Input: part model. Units: mm. Frame: model coordinates. A direction names the side the tool comes from. Give positions to 0.01 mm unless a question says otherwise; leave off trailing zeros. Loops run counter-clockwise (first coordinate to the right, second up) from the corner with the lowest first, then second, coordinate; pieces in that order, holes last. Notation, with made-up numbers: (-28.75, 65.25) - (-13.75, 65.25) arc R15 cw to (-13.75, 86.25) - close; hole circle Ø9 at (26, 39.25). An arc over 180 degrees is marked (long way). Answer as a JSON object with one key per item and string values. Group by question number.
(1) Access query for faces 1 (the flat face through (62.5, 22, 0)), 2 (the flat face through (-30, 4, 0)). Directions: +Z, -Z, +X, -X, +Y, -Y. A direction counts if a zero-diameter tool reaches every point of the face in a straight line with its end or side. Return the directions, or none.
(2) Pin query (flat end, axial travel): P1, Ø8.5, axis at x = 10, z = -4.5, coming from the +Y side; P2, Ø15, axis at x = 41.5, z = -8, coming from the +Y side. Return the tip coordinate at first contact, or that it passes through.
(3) Material intervals for L1, parallel to X at y = 7.5, z = 19.5; L2, parallel to Z at x = 12.5, y = 9.5; L3, parallel to X at y = 16, z = -3.5, sorted ascending.
(4) Section query A-A (y = 27.5). Return loops of the section in (x, z).
(5) Section query D-D (x = -30). Return loops of the section in (y, z).
(6) Section query B-B (z = 18). Return loops of the section in (x, y), plus the area to 3 significant figures.
(7) Section query C-C (x = 48). Return loops of the section in (y, z).
(8) Mould query, pull axis X, two halves, no side actions, for faces 3 (the flat face through (-62.5, 22, 0)), 4 (the flat face through (-1, 22, 23)), 5 (the flat face through (15, 8.5, 0)), 6 (the flat face through (59.5, 25, 0)). Classes: +X half, -X half, draft (parallel to the pull), parting line (faces both ways), or undercut.
```python
from build123d import *

# Parameters (mm, degrees)
SKETCH1_W           = 119
SKETCH1_H           = 40
BOSS_EXTRUDE1_DEPTH = 4
SKETCH2_W           = 125
SKETCH2_H           = 46
SKETCH2_W_2         = 119
SKETCH2_H_2         = 40
BOSS_EXTRUDE2_DEPTH = 44
SKETCH3_W           = 58.2
SKETCH3_H           = 40
BOSS_EXTRUDE3_DEPTH = 3
SKETCH4_W           = 28
SKETCH4_H           = 40
BOSS_EXTRUDE4_DEPTH = 1.5


with BuildPart() as part:
    # Sketch1 → Boss-Extrude1 (new body)
    with BuildSketch(Plane(origin=(0, 0, 0), x_dir=(1, 0, 0), z_dir=(0, 1, 0))):
        Rectangle(SKETCH1_W, SKETCH1_H)
    extrude(amount=BOSS_EXTRUDE1_DEPTH)

    # Sketch2 → Boss-Extrude2 (add)
    with BuildSketch(Plane(origin=(0, 0, 0), x_dir=(1, 0, 0), z_dir=(0, 1, 0))):
        Rectangle(SKETCH2_W, SKETCH2_H)
        Rectangle(SKETCH2_W_2, SKETCH2_H_2, mode=Mode.SUBTRACT)
    extrude(amount=BOSS_EXTRUDE2_DEPTH)

    # Sketch3 → Boss-Extrude3 (add)
    with BuildSketch(Plane(origin=(0, 4, 0), x_dir=(1, 0, 0), z_dir=(0, 1, 0))):
        with Locations((30.4, 0)):
            Rectangle(SKETCH3_W, SKETCH3_H)
    extrude(amount=BOSS_EXTRUDE3_DEPTH)

    # Sketch4 → Boss-Extrude4 (add)
    with BuildSketch(Plane(origin=(0, 7, 0), x_dir=(1, 0, 0), z_dir=(0, 1, 0))):
        with Locations((15.3, 0)):
            Rectangle(SKETCH4_W, SKETCH4_H)
    extrude(amount=BOSS_EXTRUDE4_DEPTH)


solid = part.part
```
Recorded:
{
 "1": {"face 1": "+Z, -Z, +X, +Y, -Y", "face 2": "+Y"},
 "2": {"P1": "stops at y = 8.5", "P2": "stops at y = 7"},
 "3": {"L1": "x = -62.5 to -59.5, 1.3 to 29.3, 59.5 to 62.5", "L2": "z = -23 to -20, 20 to 23", "L3": "x = -62.5 to -59.5, 59.5 to 62.5"},
 "4": {"outline": "(-62.5, -23) - (62.5, -23) - (62.5, 23) - (-62.5, 23) - close; hole (-59.5, -20) - (59.5, -20) - (59.5, 20) - (-59.5, 20) - close"},
 "5": {"outline": "(0, -23) - (44, -23) - (44, -20) - (4, -20) - (4, 20) - (44, 20) - (44, 23) - (0, 23) - close"},
 "6": {"outline": "(-62.5, 0) - (62.5, 0) - (62.5, 44) - (59.5, 44) - (59.5, 7) - (29.3, 7) - (29.3, 8.5) - (1.3, 8.5) - (1.3, 4) - (-59.5, 4) - (-59.5, 44) - (-62.5, 44) - close", "area": "957 mm^2"},
 "7": {"outline": "(0, -23) - (44, -23) - (44, -20) - (7, -20) - (7, 20) - (44, 20) - (44, 23) - (0, 23) - close"},
 "8": {"face 3": "-X half", "face 4": "draft", "face 5": "undercut", "face 6": "undercut"}
}
